```python
from build123d import *

# Parameters (mm, degrees)
ESQUISSE1_W             = 36
ESQUISSE1_H             = 26.01
ESQUISSE1_R             = 0.175
ESQUISSE1_R_2           = 0.5
ESQUISSE1_R_3           = 0.25
BOSS_EXTRU_1_DEPTH      = 1.57
ENL_V_MAT_EXTRU_1_REACH = 46.441
ESQUISSE2_R             = 1
CONG_1_R                = 2.5


with BuildPart() as part:
    # Esquisse1 → Boss.-Extru.1 (new body)
    with BuildSketch(Plane(origin=(0, 0, 0), x_dir=(-1, 0, 0), z_dir=(0, 0, -1))):
        with Locations((-18, 13.005)):
            Rectangle(ESQUISSE1_W, ESQUISSE1_H)
        with Locations(Location((-15.5, 21.5, 0), (0, 0, 180))):
            Circle(ESQUISSE1_R, mode=Mode.SUBTRACT)
        with Locations(Location((-15.5, 20, 0), (0, 0, 180))):
            Circle(ESQUISSE1_R, mode=Mode.SUBTRACT)
        with Locations(Location((-15.5, 18.5, 0), (0, 0, 180))):
            Circle(ESQUISSE1_R, mode=Mode.SUBTRACT)
        with Locations(Location((-15.5, 15.5, 0), (0, 0, 180))):
            Circle(ESQUISSE1_R, mode=Mode.SUBTRACT)
        with Locations(Location((-15.5, 17, 0), (0, 0, 180))):
            Circle(ESQUISSE1_R, mode=Mode.SUBTRACT)
        with Locations(Location((-15.5, 12.5, 0), (0, 0, 180))):
            Circle(ESQUISSE1_R, mode=Mode.SUBTRACT)
        with Locations(Location((-15.5, 14, 0), (0, 0, 180))):
            Circle(ESQUISSE1_R, mode=Mode.SUBTRACT)
        with Locations(Location((-7, 17, 0), (0, 0, 180))):
            Circle(ESQUISSE1_R_2, mode=Mode.SUBTRACT)
        with Locations(Location((-20.5, 21, 0), (0, 0, 180))):
            Circle(ESQUISSE1_R, mode=Mode.SUBTRACT)
        with Locations(Location((-20.5, 18.5, 0), (0, 0, 180))):
            Circle(ESQUISSE1_R, mode=Mode.SUBTRACT)
        with Locations(Location((-20.5, 15.5, 0), (0, 0, 180))):
            Circle(ESQUISSE1_R, mode=Mode.SUBTRACT)
        with Locations(Location((-20.5, 17, 0), (0, 0, 180))):
            Circle(ESQUISSE1_R, mode=Mode.SUBTRACT)
        with Locations(Location((-20.5, 12.5, 0), (0, 0, 180))):
            Circle(ESQUISSE1_R, mode=Mode.SUBTRACT)
        with Locations(Location((-20.5, 14, 0), (0, 0, 180))):
            Circle(ESQUISSE1_R, mode=Mode.SUBTRACT)
        with Locations(Location((-2.5, 24, 0), (0, 0, 180))):
            Circle(ESQUISSE1_R_2, mode=Mode.SUBTRACT)
        with Locations(Location((-29, 17, 0), (0, 0, 180))):
            Circle(ESQUISSE1_R_2, mode=Mode.SUBTRACT)
        with Locations(Location((-2.5, 2.5, 0), (0, 0, 180))):
            Circle(ESQUISSE1_R_2, mode=Mode.SUBTRACT)
        with Locations(Location((-33.5, 2.5, 0), (0, 0, 180))):
            Circle(ESQUISSE1_R_2, mode=Mode.SUBTRACT)
        with Locations(Location((-33.5, 24, 0), (0, 0, 180))):
            Circle(ESQUISSE1_R_2, mode=Mode.SUBTRACT)
        with Locations(Location((-10.55, 4.39, 0), (0, 0, 180))):
            Circle(ESQUISSE1_R_3, mode=Mode.SUBTRACT)
        with Locations(Location((-13.05, 4.39, 0), (0, 0, 180))):
            Circle(ESQUISSE1_R_3, mode=Mode.SUBTRACT)
        with Locations(Location((-15.55, 4.39, 0), (0, 0, 180))):
            Circle(ESQUISSE1_R_3, mode=Mode.SUBTRACT)
        with Locations(Location((-25.55, 4.39, 0), (0, 0, 180))):
            Circle(ESQUISSE1_R_3, mode=Mode.SUBTRACT)
        with Locations(Location((-19.3, 4.39, 0), (0, 0, 180))):
            Circle(ESQUISSE1_R_3, mode=Mode.SUBTRACT)
        with Locations(Location((-21.8, 4.39, 0), (0, 0, 180))):
            Circle(ESQUISSE1_R_3, mode=Mode.SUBTRACT)
        with Locations(Location((-24.3, 4.39, 0), (0, 0, 180))):
            Circle(ESQUISSE1_R_3, mode=Mode.SUBTRACT)
        with Locations(Location((-23.05, 4.39, 0), (0, 0, 180))):
            Circle(ESQUISSE1_R_3, mode=Mode.SUBTRACT)
        with Locations(Location((-20.55, 4.39, 0), (0, 0, 180))):
            Circle(ESQUISSE1_R_3, mode=Mode.SUBTRACT)
        with Locations(Location((-18.05, 4.39, 0), (0, 0, 180))):
            Circle(ESQUISSE1_R_3, mode=Mode.SUBTRACT)
        with Locations(Location((-16.8, 4.39, 0), (0, 0, 180))):
            Circle(ESQUISSE1_R_3, mode=Mode.SUBTRACT)
        with Locations(Location((-14.3, 4.39, 0), (0, 0, 180))):
            Circle(ESQUISSE1_R_3, mode=Mode.SUBTRACT)
        with Locations(Location((-11.8, 4.39, 0), (0, 0, 180))):
            Circle(ESQUISSE1_R_3, mode=Mode.SUBTRACT)
    extrude(amount=-BOSS_EXTRU_1_DEPTH)

    # Esquisse2 → Enlèv. mat.-Extru.1 (cut, up to next)
    with BuildSketch(Plane.XY.offset(1.57), mode=Mode.PRIVATE) as enl_v_mat_extru_1_sk1:
        with Locations((7, 17)):
            Circle(ESQUISSE2_R)
    enl_v_mat_extru_1_tool1 = extrude(enl_v_mat_extru_1_sk1.sketch, amount=-ENL_V_MAT_EXTRU_1_REACH, mode=Mode.PRIVATE) & part.part
    # Esquisse2 → Enlèv. mat.-Extru.1 (cut, up to next)
    with BuildSketch(Plane.XY.offset(1.57), mode=Mode.PRIVATE) as enl_v_mat_extru_1_sk2:
        with Locations((29, 17)):
            Circle(ESQUISSE2_R)
    enl_v_mat_extru_1_tool2 = extrude(enl_v_mat_extru_1_sk2.sketch, amount=-ENL_V_MAT_EXTRU_1_REACH, mode=Mode.PRIVATE) & part.part
    add(enl_v_mat_extru_1_tool1.solids().sort_by_distance((7, 17, 1.57))[0], mode=Mode.SUBTRACT)
    add(enl_v_mat_extru_1_tool2.solids().sort_by_distance((29, 17, 1.57))[0], mode=Mode.SUBTRACT)

    # Congé1
    cong_1_edges = [part.edges().sort_by_distance(p)[0] for p in [
        (0, 0, 0.785),
        (36, 0, 0.785),
    ]]
    fillet(cong_1_edges, radius=CONG_1_R)


solid = part.part
```
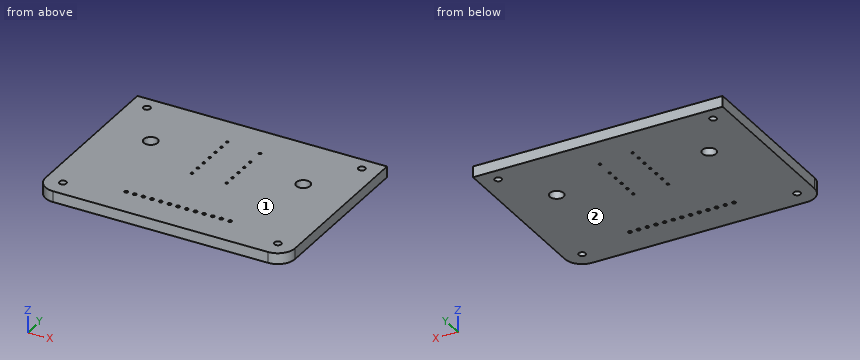
Can you work these out from the model? Positions are in its coordinate system, mm. Face numbers are marked on the shaded views. Coordinates: 2 decimals unless noted, no trailing zeros. Order: outer loops, then holes, each group sorted by start corner. A loop starts at its lowest first (then second) coordinate and runs counter-clockwise, first axis right, second up. Notation, with made-up numbers: (71, 45) -> (94, 45) arc R11 cw to (94, 58) -> close; hole circle Ø8 at (30, 4.5). An arc over 180 degrees is marked (long way). Write each question's results on one line, items separated by ' | '.
Item 1: I'm going to push a flat-ended pin straight in: pin 1 Ø1 at (x, y) = (6, 19.5) entering from -Z. Where does the tip first touch, or does it pass through?
Results are:
pin 1: z = 0
Item 2: If I drill on line 1 along Y through (x, z) = (33.5, 0.7); line 2 along X through (y, z) = (24, 0.8); line 3 along X through (y, z) = (14, 0.6) (3 decimals), over which ranges is the centre line in solid material (lowest first)?
Results are:
line 1: 0 to 2, 3 to 23.5, 24.5 to 26.01 | line 2: 0 to 2, 3 to 33, 34 to 36 | line 3: 0 to 15.325, 15.675 to 20.325, 20.675 to 36
Item 3: I want a section at A-A, the plane x = 29. Write out the boundary of the cut face in (y, z), then the cut area to 3 significant figures.
Results are:
outline: (0, 0) -> (16, 0) -> (16, 1.57) -> (0, 1.57) -> close; (18, 0) -> (26.01, 0) -> (26.01, 1.57) -> (18, 1.57) -> close | area: 37.7 mm²
Item 4: I want a section at B-B, the plane z = 0.3. Count the separate pieces of the cut face and the enclosed holes in it, then the cut area to 3 significant figures.
Results are:
separate pieces: 1 | enclosed holes: 32 | area: 920 mm²
Item 5: If we mould it in two halves opening along Z, with no side actions, what happens to the marked faces 1 and 2? For each: +Z half, -Z half, draft (parallel to the pull), parting line (faces both ways), or undercut.
Results are:
face 1: +Z half | face 2: -Z half
